Here's how the part is built. I have some questions about the finished solid (model axes, mm). A direction names the side the tool comes from. Round coordinates to 2 decimals unless told otherwise and drop trailing zeros. Loops run counter-clockwise (first coordinate to the right, second up) from the corner with the lowest first, then second, coordinate; pieces in that order, holes last. Notation, with made-up numbers: M 50.5,-10 L 66.5,-10 A28 cw 66.5,15 Z; hole C 76.5,54 d11. An arc over 180 degrees is marked long. Put each result on its own line as item: value. Start each with the question number.
```python
from build123d import *

# Parameters (mm, degrees)
F0_W          = 25.4
F0_H          = 127
F1_DEPTH      = 25.4
F2_DEPTH      = 25.4
F2_DEPTH_BACK = 25.4
F3_R          = 5.08


with BuildPart() as f1:
    # F0 (on Front) → F1 (new body, symmetric)
    with BuildSketch(Plane.XZ):
        with Locations((-12.7, 63.5)):
            Rectangle(F0_W, F0_H)
    extrude(amount=F1_DEPTH, both=True)

    # F0 (on Front) → F2 (join, two sides)
    with BuildSketch(Plane.XZ) as f2_sk:
        Polygon((91.7868316174, 0), (0, 0), (-25.4, 0), (-25.4, -22.6269382983), (91.7868316174, -22.6269382983), align=None)
    extrude(amount=F2_DEPTH)
    extrude(f2_sk.sketch, amount=-F2_DEPTH_BACK)

    # F3
    f3_edges = [f1.edges().sort_by_distance(p)[0] for p in [
        (0, 0, 0),
    ]]
    fillet(f3_edges, radius=F3_R)


solid = f1.part
```
1) Suppose I cut it at B-B (x = 7.5). Write out the boundary of the cut face in (y, z).
2) I'm going to push flat-ended pins straight in: P1, Ø2, axis at x = 69, y = 11, coming from the +Z side; P2, Ø1.5, axis at y = -2, z = 29, coming from the +X side. Where does each tip first touch, or does it pass through?
3) If I drill on probe 1 along Z at (x, y) = (69, 20); probe 2 along X at (y, z) = (6, 17.5); probe 3 along X at (y, z) = (-2, 4), over which ranges is the centre line in solid material (lowest first)? Write a range as from..to.
4) On a 3-axis mill with a long thin cutter (end or side, diameter ignored), from which of +Z, -Z, +X, -X, +Y, -Y can I reach the whole of each face in a straight line? I mean faces 1 (the face through (-2, 25.4, 36)), 2 (the face through (0, 0, 65)). Say none if no direction works.
5) Suppose I cut it at A-A (y = 22.5). Write out the boundary of the cut face in (x, z).
6) Suppose I cut it at C-C (z = 83.5). Write out the boundary of the cut face in (x, y).
Results are:
1. outline: M -25.4,-22.63 L 25.4,-22.63 L 25.4,0 L -25.4,0 Z
2. P1: z = 0
2. P2: x = 0
3. probe 1: -22.63..0
3. probe 2: -25.4..0
3. probe 3: -25.4..0.12
4. face 1: +Z, -Z, +X, -X, +Y
4. face 2: +Z, +X, +Y, -Y
5. outline: M -25.4,-22.63 L 91.79,-22.63 L 91.79,0 L 5.08,0 A5.08 cw 0,5.08 L 0,127 L -25.4,127 Z
6. outline: M -25.4,-25.4 L 0,-25.4 L 0,25.4 L -25.4,25.4 Z
